The listing builds one solid part. Answer for the finished solid, in the listing's coordinates (mm). A direction names the side the tool comes from. Round coordinates to 2 decimals unless told otherwise and drop trailing zeros. Loops run counter-clockwise (first coordinate to the right, second up) from the corner with the lowest first, then second, coordinate; pieces in that order, holes last. Notation, with made-up numbers: (89.5, 53) -> (107.5, 53) arc R18 ccw to (107.5, 73) -> close; hole circle Ø9 at (-32.75, -13). An arc over 180 degrees is marked (long way). Answer in a Markdown table with one row per item. Add a question column.
Autodesk Inventor part; units mm, degrees
ref_plane "YZ Plane" through (0, 0, 0) normal (1, 0, 0) x (0, 1, 0)
ref_plane "XZ Plane" through (0, 0, 0) normal (0, 1, 0) x (-1, 0, 0)
ref_plane "XY Plane" through (0, 0, 0) normal (0, 0, 1) x (1, 0, 0)
ref_plane "Work Plane1" through (0, 0, -8) normal (0, 0, 1) x (1, 0, 0)
sketch "Sketch1" plane through (0, 0, -8) normal (0, 0, 1) x (1, 0, 0)
  circle A0 centre (0, 0) radius 13.09
  circle A1 centre (0, 0) radius 10
  circle A2 centre (0, 0) radius 13.09
  circle A3 centre (0, 0) radius 10.3
  circle A4 centre (0, 0) radius 14.3
  line L0 (-7.8163, 11.9748) -> (-4.2157, 15.9521) construction
  line L1 (-4.2157, 15.9521) -> (-9.9494, 19.4831) construction
  spline S0 degree 2 poles (-7.8163, 11.9748) (-4.2157, 15.9521) (-9.9494, 19.4831) knots 1 1 1 2 2 2
  line L2 (-9.9494, 19.4831) -> (-9.2931, 20.5487)
  line L3 (-9.3147, 20.5137) -> (-3.3697, 16.8527) construction
  line L4 (-3.3697, 16.8527) -> (-4.8153, 13.4649) construction
  spline S1 degree 2 poles (-9.3147, 20.5137) (-3.3697, 16.8527) (-4.8153, 13.4649) knots 1 1 1 2 2 2
  line L5 (-4.8153, 13.4649) -> (-7.5493, 7.007)
  line L6 (0, 0) -> (0, 1.6434)
  line L7 (7.8163, 11.9748) -> (4.2157, 15.9521) construction
  line L8 (4.2157, 15.9521) -> (9.9494, 19.4831) construction
  spline S2 degree 2 poles (7.8163, 11.9748) (4.2157, 15.9521) (9.9494, 19.4831) knots 1 1 1 2 2 2
  line L9 (9.9494, 19.4831) -> (9.2931, 20.5487)
  line L10 (9.3147, 20.5137) -> (3.3697, 16.8527) construction
  line L11 (3.3697, 16.8527) -> (4.8153, 13.4649) construction
  spline S3 degree 2 poles (9.3147, 20.5137) (3.3697, 16.8527) (4.8153, 13.4649) knots 1 1 1 2 2 2
  line L12 (4.8153, 13.4649) -> (7.5493, 7.007)
  point P0 (0, 0)
  point P1 (4.8153, 13.4649)
  point P2 (7.5493, 7.007)
  point P3 (-4.8153, 13.4649)
  point P4 (7.8163, 11.9748)
  point P5 (4.8153, 13.4649)
  dimension "d0" = 0.3
  dimension "d1" = 4
extrude "Extrusion1" add sketch "Sketch1" along normal blind 2 contours A0 L5 A3 L12 | A0 L12 A4 L5 | S3 L9 S2 A4 | A4 S0 L2 S1 picked at (-7.0541, 9.7176) picked at (13.6381, 2.1556)
properties part number "axle_cap_3DPrint"
Item 1: Section A-A, the plane y = 0 is taken. Write down the section's boundary in (x, z), and give its area (3 significant figures).
Item 2: Section B-B, the plane x = 0 is taken. Write down the section's boundary in (y, z), and give its area (3 significant figures).
Item 3: Consider L1, parallel to X at y = 0, z = -7.55; L2, parallel to X at y = 3, z = -6.65; L3, parallel to Y at x = 0, z = -6.7. Determine where each line is inside the solid, lowest interval first. Write a range as from..to.
Item 4: Section C-C, the plane x = 3 is taken. Write down the section's boundary in (y, z).
Item 5: For faces 5 (the flat face through (9.636, 19.991, -7.014)), 6 (the flat face through (6.163, 10.281, -7.014)), determine the directions among +Z, -Z, +X, -X, +Y, -Y from which every point of the face is accessible in a straight line to the end or side of a thin tool.
Item 6: The mould has two halves that part along Y. Classify faces 1 (the flat face through (4, -10, -6)), 2 (the cylindrical face through (0.334, -10.295, -7.014)), 3 (the flat face through (-9.636, 19.991, -7.014)), 4 (the flat face through (-6.163, 10.281, -7.014)): +Y half, -Y half, draft (parallel to the pull), parting line (faces both ways), or undercut.
Item 7: Flat-ended cylindrical pins translate along their axes: P1, Ø6, axis at x = -3, y = 7.5, coming from the +Z side; P2, Ø1, axis at y = -7, z = -6.5, coming from the +X side. Find the tip coordinate at first contact, or state that the pin passes through.
Here are the results:
| question | item | result |
|---|---|---|
| 1 | outline | (-14.3, -8) -> (-10.3, -8) -> (-10.3, -6) -> (-14.3, -6) -> close; (10.3, -8) -> (14.3, -8) -> (14.3, -6) -> (10.3, -6) -> close |
| 1 | area | 16.0 mm² |
| 2 | outline | (-14.3, -8) -> (-10.3, -8) -> (-10.3, -6) -> (-14.3, -6) -> close |
| 2 | area | 8.00 mm² |
| 3 | L1 | x = -14.3..-10.3, 10.3..14.3 |
| 3 | L2 | x = -13.98..-9.85, 9.85..13.98 |
| 3 | L3 | y = -14.3..-10.3 |
| 4 | outline | (-13.98, -8) -> (-9.85, -8) -> (-9.85, -6) -> (-13.98, -6) -> close |
| 5 | face 5 | +Z, -Z, +X, +Y |
| 5 | face 6 | +Z, -Z |
| 6 | face 1 | draft |
| 6 | face 2 | undercut |
| 6 | face 3 | +Y half |
| 6 | face 4 | undercut |
| 7 | P1 | passes through |
| 7 | P2 | stops at x = 12.74 |
